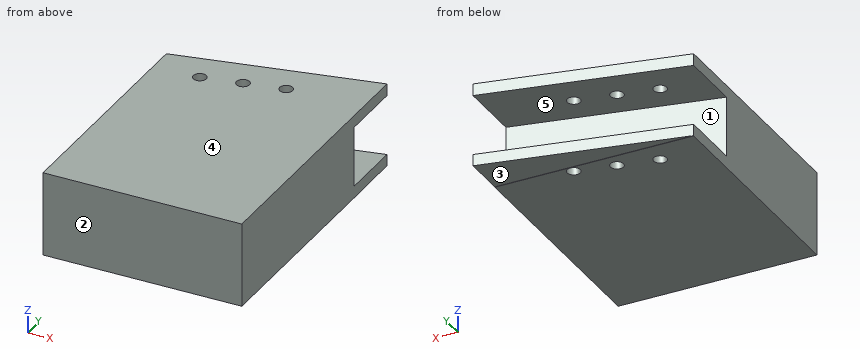
```python
from build123d import *

# Parameters (mm, degrees)
SKETCH_1_W          = 50
SKETCH_1_H          = 60
EXTRUDE_1_DEPTH     = 10.6
EXTRUDE_2_DEPTH     = 3
EXTRUDE_START       = -18.1
EXTRUDE_3_DEPTH     = 3
SWEEP_START         = -7.6
SWEEP_1_DEPTH       = 15.2
SKETCH_4_R          = 1.65
CUT_EXTRUDE_1_DEPTH = 3


# Read off the part's stored shape, not the designer's step: the sweep step
with BuildPart() as part:
    # Sketch 1 → Extrude 1 (new, symmetric)
    with BuildSketch(Plane.XY):
        Rectangle(SKETCH_1_W, SKETCH_1_H)
    extrude(amount=EXTRUDE_1_DEPTH, both=True)

    # Sketch 2 → Extrude 2 (add)
    with BuildSketch(Plane.XY.offset(10.6)):
        Polygon((-25, 30), (25, 40.627828084), (25, 30), align=None)
    extrude(amount=-EXTRUDE_2_DEPTH)

    # Sketch 2_2 → Extrude 3 (add)
    with BuildSketch(Plane.XY.offset(10.6).offset(EXTRUDE_START)):
        Polygon((-25, 30), (25, 40.627828084), (25, 30), align=None)
    extrude(amount=-EXTRUDE_3_DEPTH)

    # Sweep 1 outline → Sweep 1 (cut)
    with BuildSketch(Plane.XY.offset(SWEEP_START)):
        Polygon((-25, 30), (-25, 14), (25, 24.627828084), (25, 40.627828084), align=None)
    extrude(amount=SWEEP_1_DEPTH, mode=Mode.SUBTRACT)

    # Sketch 4 → Cut-Extrude 1 (cut)
    with BuildSketch(Plane.XY.offset(-7.6)):
        with Locations((-13.523968529, 24.106860253)):
            Circle(SKETCH_4_R)
        with Locations((-3.742492522, 26.185977161)):
            Circle(SKETCH_4_R)
        with Locations((6.038983485, 28.265094069)):
            Circle(SKETCH_4_R)
    cut_extrude_1 = extrude(amount=-CUT_EXTRUDE_1_DEPTH, mode=Mode.SUBTRACT)

    # Mirror 1: Cut-Extrude 1 across plane
    add(cut_extrude_1.mirror(Plane.XY), mode=Mode.SUBTRACT)


solid = part.part
```
Build history of the part. All positions in model axes, mm. Face numbers are marked on the shaded views. A direction names the side the tool comes from. Round coordinates to 2 decimals unless told otherwise and drop trailing zeros. Write each loop counter-clockwise with the first axis right and the second up, starting at its lowest first coordinate (ties: lowest second). Pieces come first, ordered by that corner, then holes. Notation, with made-up numbers: (15, 3.25) - (47, 3.25) arc R19 ccw to (47, 40.25) - close; hole circle Ø6 at (31, -4.75). An arc over 180 degrees is marked (long way). Answer as CSV lines item,"result".
Q1. Cut at D-D (z = -2.5). Write the cut outline in (x, y), and give its area (3 significant figures).
Report:
outline,"(-25, -30) - (25, -30) - (25, 24.63) - (-25, 14) - close"
area,"2,470 mm^2"
Q2. Drill centre lines: probe 1 along Z at (x, y) = (-18.5, 26); probe 2 along Y at (x, z) = (7.5, 9.5); probe 3 along Y at (x, z) = (-13.5, -9.5). Where is each one in solid material? Low to high. Write a range as [from, to].
Report:
probe 1,"z = [-10.6, -7.6], [7.6, 10.6]"
probe 2,"y = [-30, 27.5], [29.03, 36.91]"
probe 3,"y = [-30, 22.46], [25.76, 32.44]"
Q3. Tool access for the marked faces 4 and 5: list every direction of +Z, -Z, +X, -X, +Y, -Y with a clear straight run to the whole face (end or side of a thin tool).
Report:
face 4,"+Z, +X, -X, +Y, -Y"
face 5,"-X, +Y"
Q4. Drop flat-ended pins along their axis: pin 1 (8.5 mm diameter, centred on x = 4.5, y = 36.5, fed in from -Z); pin 2 (6 mm diameter, centred on x = -8, z = -4, fed in from +Y). Give the stop position or say it passes through.
Report:
pin 1,"stops at z = -10.5"
pin 2,"stops at y = 18.25"
Q5. Cut at C-C (y = 20). Write the cut outline in (x, z), and give its area (3 significant figures).
Report:
outline,"(-25, -10.6) - (25, -10.6) - (25, 10.6) - (-25, 10.6) - (-25, 7.6) - (3.23, 7.6) - (3.23, -7.6) - (-25, -7.6) - close"
area,"631 mm^2"
Q6. Cut at B-B (x = -19.5). Write the cut outline in (y, z), and give its area (3 significant figures).
Report:
outline,"(-30, -10.6) - (30, -10.6) - (30, -10.5) - (31.17, -10.5) - (31.17, -7.6) - (15.17, -7.6) - (15.17, 7.6) - (31.17, 7.6) - (31.17, 10.6) - (-30, 10.6) - close"
area,"1,050 mm^2"
Q7. Pull direction Z, two halves, no side cores. Call the marked faces 1, 2 and 3: +Z half, -Z half, draft (parallel to the pull), parting line (faces both ways), or undercut.
Report:
face 1,"undercut"
face 2,"draft"
face 3,"-Z half"
Q8. Cut at A-A (z = -8.75). Write the cut outline in (x, y), and give its area (3 significant figures).
Report:
outline,"(-25, -30) - (25, -30) - (25, 40.63) - (-25, 30) - close; hole circle Ø3.3 at (-13.52, 24.11); hole circle Ø3.3 at (-3.74, 26.19); hole circle Ø3.3 at (6.04, 28.27)"
area,"3,240 mm^2"
